Could you check a few things on this model? Use its own coordinates, in mm. Face numbers are marked on the shaded views. A direction names the side the tool comes from. Round coordinates to 2 decimals unless told otherwise and drop trailing zeros. Loops run counter-clockwise (first coordinate to the right, second up) from the corner with the lowest first, then second, coordinate; pieces in that order, holes last. Notation, with made-up numbers: (65.5, -16) -> (100.5, -16) arc R17 ccw to (100.5, 14) -> close; hole circle Ø8 at (74, 46.5). An arc over 180 degrees is marked (long way). Put each result on its own line as item: value. Start each with the question number.
1. Imagine slicing it at A-A, the plane y = 47. Please give me the cut outline in (x, z).
2. Imagine slicing it at C-C, the plane z = -8. Please give me the cut outline in (x, y), and give its area (3 significant figures).
3. I need wall thicknesses on line 1 (Y direction, x = 0, z = 1.95); line 2 (Z direction, x = 0, y = 1.2); line 3 (Z direction, x = -1.5, y = 47.5). Which ranges of each line are inside material? Lowest first, please. Write a range as [from, to].
4. Imagine slicing it at D-D, the plane x = -3. Please give me the cut outline in (y, z), and give its area (3 significant figures).
5. Which directions (+Z, -Z, +X, -X, +Y, -Y) give clear straight access to the entire face, cutting with the end or side of a thin tool? Please do the marked faces 1, 2 and 3.
6. Imagine slicing it at B-B, the plane x = 0. Count the separate pieces of the cut face and the enclosed holes in it, and give its area (3 significant figures).
7. I'm going to push flat-ended pins straight in: P1, Ø2, axis at x = 0, y = 38, coming from the +Z side; P2, Ø1.6, axis at x = -1, z = 0, coming from the +Y side; P3, Ø1, axis at x = -2, y = 31.5, coming from the -Z side. Where does each tip first touch, or does it pass through?
Autodesk Inventor part; units mm, degrees
ref_plane "YZ Plane" through (0, 0, 0) normal (1, 0, 0) x (0, 1, 0)
ref_plane "XZ Plane" through (0, 0, 0) normal (0, 1, 0) x (-1, 0, 0)
ref_plane "XY Plane" through (0, 0, 0) normal (0, 0, 1) x (1, 0, 0)
sketch "Sketch1" plane through (0, 0, 0) normal (0, 1, 0) x (-1, 0, 0)
  line L0 (-3.5, 2.5) -> (3.5, 2.5)
  line L1 (3.5, 2.5) -> (3.5, -2.5)
  line L2 (3.5, -2.5) -> (-3.5, -2.5)
  line L3 (-3.5, -2.5) -> (-3.5, 2.5)
  line L4 (-3.5, 2.5) -> (3.5, -2.5) construction
  line L5 (3.5, 2.5) -> (-3.5, -2.5) construction
  point P0 (0, 0)
  dimension "d0" = 5
  dimension "d1" = 7
extrude "Extrusion1" add sketch "Sketch1" along normal blind 50
sketch "Sketch2" plane through (0, 50, 0) normal (0, 1, 0) x (1, 0, 0)
  line L0 (-3.5, -2.5) -> (3.5, -2.5)
  line L1 (3.5, -2.5) -> (3.5, 2.5)
  line L2 (3.5, 2.5) -> (-3.5, 2.5)
  line L3 (-3.5, 2.5) -> (-3.5, -2.5)
  line L4 (-3.5, -1) -> (3.5, -1)
  line L5 (3.5, -1) -> (3.5, 1)
  line L6 (3.5, 1) -> (-3.5, 1)
  line L7 (-3.5, 1) -> (-3.5, -1)
  point P0 (0, 0)
  dimension "d4" = 1.5
  dimension "d5" = 1.5
extrude "Extrusion2" cut sketch "Sketch2" against normal blind 6 contours L3 L6 L1 L4
sketch "Sketch3" plane through (3.5, 0, -2.5) normal (0, 0, -1) x (-1, 0, 0)
  line L0 (7, 0) -> (7, 50)
  line L1 (0, 50) -> (7, 50)
  circle A0 centre (3.5, 47) radius 1
  point P0 (3.5, 0)
  dimension "d8" = 2
  dimension "d9" = 3
  dimension "d10" = 3.5
extrude "Extrusion3" cut sketch "Sketch3" against normal through all
sketch "Sketch4" plane through (3.5, 0, 2.5) normal (1, 0, 0) x (0, 0, -1)
  line L0 (5, 0) -> (5, 50)
  line L1 (0, 0) -> (0, 50)
  line L2 (0, 0) -> (5, 0)
  circle A0 centre (2.5, 0) radius 4
  line L3 (8.1, 0) -> (-3.1, 0)
  dimension "d21" = 8
extrude "Extrusion4" cut sketch "Sketch4" against normal through all
sketch "Sketch6" plane through (3.5, 44, -1) normal (1, 0, 0) x (0, 0, -1)
  arc A0 (1.5, -40.8775) -> (-3.5, -40.8775) centre (-1, -44) ccw construction
  line L0 (1.5, -40.8775) -> (1.5, 6)
  line L1 (-3.5, -40.8775) -> (-3.5, 6)
  arc A1 (-3.5, -40.8775) -> (-5, -44) centre (-1, -44) ccw
  line L2 (4.6, -44) -> (-6.6, -44)
  line L3 (-15.2174, -44) -> (-5, -44) construction
  arc A2 (1.5, -40.8775) -> (-3.5, -40.8775) centre (-1, -44) ccw
  arc A3 (-5, -44) -> (3, -44) centre (-1, -44) ccw construction
  arc A4 (3, -44) -> (1.5, -40.8775) centre (-1, -44) ccw
  line L4 (-3.5, -37.8775) -> (-6.53, -42)
  line L5 (-1, -58.8) -> (-1, 16.8)
  line L6 (-4.4641, -42) -> (-6.53, -42) construction
  line L7 (-12.4641, -42) -> (-12.4641, -44)
  line L8 (-12.4641, -44) -> (-5, -44)
  line L9 (-4.4641, -44) -> (-4.4641, -42) construction
  line L10 (-6.53, -42) -> (-12.4641, -42)
  line L11 (-6.53, -42) -> (-8, -44) construction
  line L12 (-5, -44) -> (17.7359, -44) construction
  line L13 (-5, -44) -> (-4.4641, -44) construction
  line L14 (1.5, -37.8775) -> (4.53, -42)
  line L15 (10.4641, -42) -> (10.4641, -44)
  line L16 (10.4641, -44) -> (3, -44)
  line L17 (4.53, -42) -> (10.4641, -42)
  line L18 (1.5, -37.8775) -> (-3.5, -37.8775)
  dimension "d26" = 3
  dimension "d27" = 3
  dimension "d28" = 8
  dimension "d29" = 2
extrude "Extrusion5" add sketch "Sketch6" against normal blind 7 contours A2 L5 L18 L0 | L0 L14 L17 L15 L16 L2 A4 | A2 L1 L18 L5 | A1 L2 L8 L7 L10 L4 L1
sketch "Sketch7" plane through (3.5, 2, 11.4641) normal (0, 1, 0) x (1, 0, 0)
  line L0 (-7, 0) -> (-7, 5.9341)
  line L1 (0, 0) -> (-7, 0)
  circle A0 centre (-3.5, 3) radius 1
  circle A1 centre (-3.5, 19.9282) radius 1
  line L2 (-7, 16.9941) -> (-7, 22.9282)
  line L3 (0, 22.9282) -> (-7, 22.9282)
  point P0 (-3.5, 11.4641)
  dimension "d32" = 2
  dimension "d33" = 3
  dimension "d34" = 3.5
  dimension "d35" = 3.5
  dimension "d36" = 3
  dimension "d37" = 2
extrude "Extrusion6" cut sketch "Sketch7" against normal through all
properties part number "LD_holder_p5"
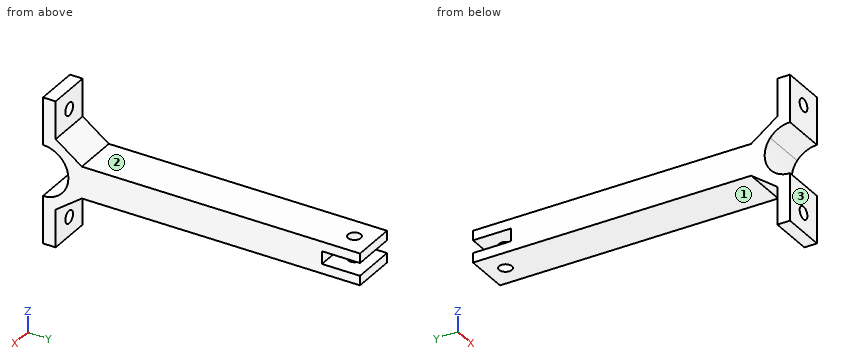
Entries:
1. outline: (-3.5, -2.5) -> (-1, -2.5) -> (-1, -1) -> (-3.5, -1) -> close; (-3.5, 1) -> (-1, 1) -> (-1, 2.5) -> (-3.5, 2.5) -> close; (1, -2.5) -> (3.5, -2.5) -> (3.5, -1) -> (1, -1) -> close; (1, 1) -> (3.5, 1) -> (3.5, 2.5) -> (1, 2.5) -> close
2. outline: (-3.5, 0) -> (-0.89, 0) -> (-0.89, 2) -> (-3.5, 2) -> close; (0.89, 0) -> (3.5, 0) -> (3.5, 2) -> (0.89, 2) -> close
2. area: 10.5 mm^2
3. line 1: [3.49, 46], [48, 50]
3. line 2: [-11.46, -9.46], [-7.46, -3.82], [3.82, 7.46], [9.46, 11.46]
3. line 3: [-2.5, -1], [1, 2.5]
4. outline: (0, -11.46) -> (2, -11.46) -> (2, -5.53) -> (6.12, -2.5) -> (50, -2.5) -> (50, -1) -> (44, -1) -> (44, 1) -> (50, 1) -> (50, 2.5) -> (6.12, 2.5) -> (2, 5.53) -> (2, 11.46) -> (0, 11.46) -> (0, 4) arc R4 cw to (3.12, 2.5) arc R4 cw to (3.12, -2.5) arc R4 cw to (0, -4) -> close
4. area: 261 mm^2
5. face 1: -Z, +X, -X, +Y
5. face 2: +Z, +X, -X, +Y
5. face 3: +Z, -Z, +X, -X, -Y
6. separate pieces: 5
6. enclosed holes: 0
6. area: 247 mm^2
7. P1: z = 2.5
7. P2: y = 44
7. P3: z = -2.5
